CAD build for the part. Positions are in the model's coordinates, mm. Round coordinates to 2 decimals unless told otherwise and drop trailing zeros. Write each loop counter-clockwise with the first axis right and the second up, starting at its lowest first coordinate (ties: lowest second). Pieces come first, ordered by that corner, then holes. Notation, with made-up numbers: (72.25, 48.5) -> (88.25, 48.5) arc R19 ccw to (88.25, 64.5) -> close; hole circle Ø7 at (83, -33). An arc over 180 degrees is marked (long way). Answer in a Markdown table with one row per item. Add a question column.
```python
from build123d import *

# Parameters (mm, degrees)
F1_DEPTH = 0.635
F2_R     = 0.635
F3_DEPTH = 1.27
F4_R     = 1.27


with BuildPart() as f1:
    # F0 (on Front) → F1 (new body, symmetric)
    with BuildSketch(Plane.XZ):
        with BuildLine():
            Line((-29.324013, 0), (0, 0))
            Line((0, 0), (-14.208709, 77.572884))
            ThreePointArc((-14.208709, 77.572884), (-22.393281, 83.788762), (-29.324013, 76.2))
            Line((-29.324013, 76.2), (-29.324013, 0))
        make_face()
    extrude(amount=F1_DEPTH, both=True)

    # F2 (on face) → F3 (cut, through all)
    with BuildSketch(Plane.XZ.offset(0.635)):
        with Locations((-21.704013, 76.2)):
            Circle(F2_R)
    extrude(amount=-F3_DEPTH, mode=Mode.SUBTRACT)

    # F4
    f4_edges = [f1.edges().sort_by_distance(p)[0] for p in [
        (-29.324013, 0, 0),
        (0, 0, 0),
    ]]
    fillet(f4_edges, radius=F4_R)


solid = f1.part
```
Item 1: Saw through at A-A on y = 0.4. Give the cut face in (x, z) (3 decimals).
Item 2: Drill centre lines: probe 1 along X at (y, z) = (-0.4, 76.2); probe 2 along Z at (x, y) = (-23, -0.35); probe 3 along Z at (x, y) = (-26.5, 0.15). Where is each one in solid material? Low to high.
Item 3: Saw through at B-B on x = -15. Give the cut face in (y, z) (3 decimals), then the cut area to 3 significant figures.
Item 4: Saw through at C-C on z = 12.5. Give the cut face in (x, y) (3 decimals).
Recorded:
| question | item | result |
|---|---|---|
| 1 | outline | (-29.324, 1.27) arc R1.27 ccw to (-28.054, 0) -> (-1.524, 0) arc R1.27 ccw to (-0.275, 1.499) -> (-14.209, 77.573) arc R7.62 ccw to (-29.324, 76.2) -> close; hole circle Ø1.27 at (-21.704, 76.2) |
| 2 | probe 1 | -29.32 to -22.34, -21.07 to -13.96 |
| 2 | probe 2 | 0 to 83.71 |
| 2 | probe 3 | 0 to 82.12 |
| 3 | outline | (-0.635, 0) -> (0.635, 0) -> (0.635, 79.822) -> (-0.635, 79.822) -> close |
| 3 | area | 101 mm2 |
| 4 | outline | (-29.324, -0.635) -> (-2.29, -0.635) -> (-2.29, 0.635) -> (-29.324, 0.635) -> close |
